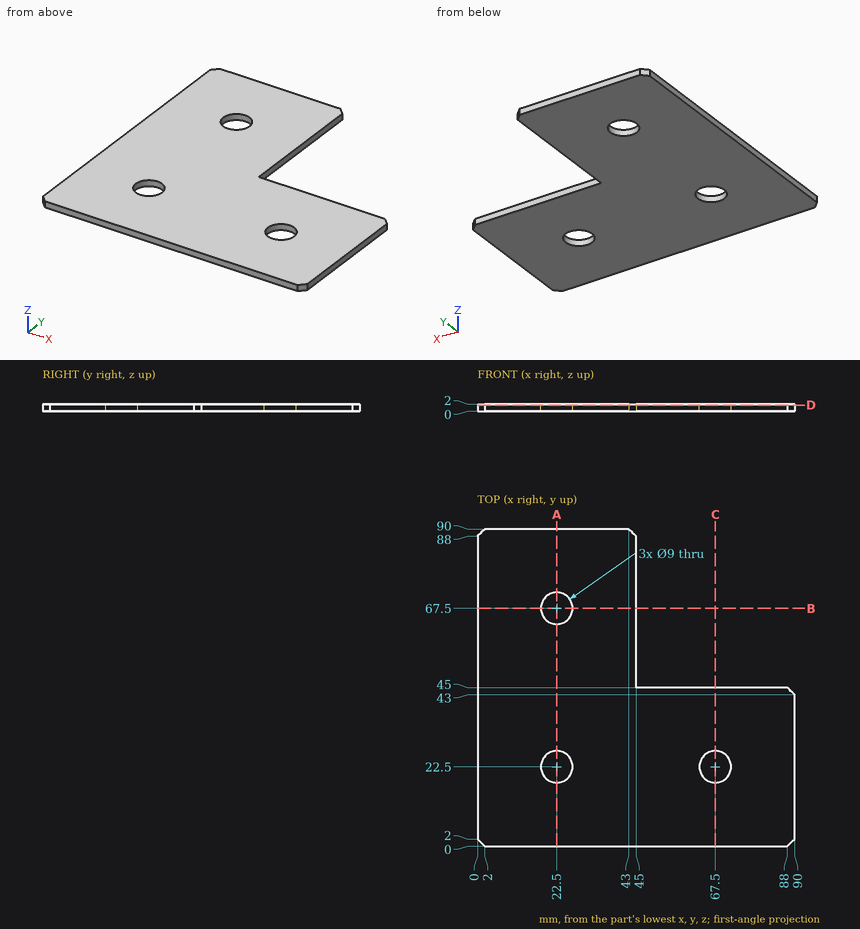
The figure shows three views and two pictorial views of one solid part (mm, origin at its lowest corner). Answer the questions. Give positions to 0.01 mm unless a question says otherwise; leave off trailing zeros. Order: outer loops, then holes, each group sorted by start corner. A loop starts at its lowest first (then second) coordinate and runs counter-clockwise, first axis right, second up. Notation, with made-up numbers: M -16.75,11 L -2.75,11 A20 ccw -2.75,35 Z; hole C -27.5,60 d11. An arc over 180 degrees is marked long. Return JSON: item names as keys, results as strings.
1) Each of these flat-tipped pins is pushed along its axis until it touches: pin 1 (1 mm diameter, centred on x = 61, z = 0.5, fed in from +Y); pin 2 (11.5 mm diameter, centred on x = 67.5, y = 22.5, fed in from -Z). Where does it stop, or does it pass through?
Resolved:
{"pin 1": "y = 45", "pin 2": "z = 0"}
2) Section D-D, the plane z = 1.7 is taken. Write down the section's boundary in (x, y), plus the area to 3 significant figures.
Resolved:
{"outline": "M 0,2 L 2,0 L 88,0 L 90,2 L 90,43 L 88,45 L 45,45 L 45,88 L 43,90 L 2,90 L 0,88 Z; hole C 22.5,22.5 d9; hole C 22.5,67.5 d9; hole C 67.5,22.5 d9", "area": "5,870 mm^2"}
3) Section A-A, the plane x = 22.5 is taken. Write down the section's boundary in (y, z).
Resolved:
{"outline": "M 0,0 L 18,0 L 18,2 L 0,2 Z; M 27,0 L 63,0 L 63,2 L 27,2 Z; M 72,0 L 90,0 L 90,2 L 72,2 Z"}
4) Section B-B, the plane y = 67.5 is taken. Write down the section's boundary in (x, z), plus the area to 3 significant figures.
Resolved:
{"outline": "M 0,0 L 18,0 L 18,2 L 0,2 Z; M 27,0 L 45,0 L 45,2 L 27,2 Z", "area": "72.0 mm^2"}
5) Straight lines are drawn through the part: line 1 along X through (y, z) = (22.5, 0.2); line 2 along Y through (x, z) = (67.5, 0.6). For each, find the intervals that lie inside material, in ascending order. Write a range as [from, to].
Resolved:
{"line 1": "[0, 18], [27, 63], [72, 90]", "line 2": "[0, 18], [27, 45]"}
